from build123d import *

# Parameters (mm, degrees)
SKETCH_2_W                       = 64.02174429
SKETCH_2_H                       = 9.248919907
CUT_EXTRUDE_1_DEPTH              = 49
HOLE_WIZARD_M4_2_D               = 3.3
HOLE_WIZARD_M4_2_DEPTH           = 5.5
HOLE_WIZARD_M4_2_TIP             = 0.991420021
HOLE_WIZARD_M6_2_D               = 5
HOLE_WIZARD_M6_2_DEPTH           = 5.5
HOLE_WIZARD_M6_2_TIP             = 1.502151548
HOLE_WIZARD_M4_3_D               = 3.3
HOLE_WIZARD_M4_3_DEPTH           = 13.4
HOLE_WIZARD_M4_3_TIP             = 0.991420021
HOLE_WIZARD_M4_3_ON_FACE_2_D     = 3.3
HOLE_WIZARD_M4_3_ON_FACE_2_DEPTH = 13.4
HOLE_WIZARD_M4_3_ON_FACE_2_TIP   = 0.991420021


with BuildPart() as part:
    # 草图1 → 旋转1 (revolve)
    with BuildSketch(Plane(origin=(0, 0, 0), x_dir=(1, 0, 0), z_dir=(0, 1, 0)), mode=Mode.PRIVATE) as revolve_1_sk:
        Polygon((34.5, 7.5), (34.5, -7.5), (25.4, -7.5), (25.4, -4), (26.5, -4), (26.5, 4), (25.4, 4), (25.4, 7.5), align=None)
    revolve(revolve_1_sk.sketch.rotate(Axis((0, 0, -31.9390681), (0, 0, 1)), 180), axis=Axis((0, 0, -31.9390681), (0, 0, 1)))  # turned: the seam where the file's is

    # 草图2 → 切除-拉伸1 (cut)
    with BuildSketch(Plane.XY.offset(7.5)):
        with Locations((-1.141100508, 38.424459954)):
            Rectangle(SKETCH_2_W, SKETCH_2_H)
        with Locations((-1.141100508, -38.424459954)):
            Rectangle(SKETCH_2_W, SKETCH_2_H)
    extrude(amount=-CUT_EXTRUDE_1_DEPTH, mode=Mode.SUBTRACT)

    # M4 螺纹孔2
    with Locations(Plane(origin=(0, 33.8, 0), x_dir=(1, 0, 0), z_dir=(0, 1, 0))):
        with Locations((0, 0)):
            Hole(HOLE_WIZARD_M4_2_D / 2, depth=HOLE_WIZARD_M4_2_DEPTH)
            with Locations((0, 0, -(HOLE_WIZARD_M4_2_DEPTH + HOLE_WIZARD_M4_2_TIP / 2))):  # 118° drill point
                Cone(0, HOLE_WIZARD_M4_2_D / 2, HOLE_WIZARD_M4_2_TIP, mode=Mode.SUBTRACT)

    # M6 螺纹孔2
    with Locations(Plane(origin=(0, -33.8, 0), x_dir=(-1, 0, 0), z_dir=(0, -1, 0))):
        with Locations((0, 0)):
            Hole(HOLE_WIZARD_M6_2_D / 2, depth=HOLE_WIZARD_M6_2_DEPTH)
            with Locations((0, 0, -(HOLE_WIZARD_M6_2_DEPTH + HOLE_WIZARD_M6_2_TIP / 2))):  # 118° drill point
                Cone(0, HOLE_WIZARD_M6_2_D / 2, HOLE_WIZARD_M6_2_TIP, mode=Mode.SUBTRACT)

    # M4 螺纹孔3
    with Locations(Plane(origin=(29.877876431, 17.25, 0), x_dir=(-0.5, 0.866025404, 0), z_dir=(0.866025404, 0.5, 0))):
        with Locations((0, 0)):
            Hole(HOLE_WIZARD_M4_3_D / 2, depth=HOLE_WIZARD_M4_3_DEPTH)
            with Locations((0, 0, -(HOLE_WIZARD_M4_3_DEPTH + HOLE_WIZARD_M4_3_TIP / 2))):  # 118° drill point
                Cone(0, HOLE_WIZARD_M4_3_D / 2, HOLE_WIZARD_M4_3_TIP, mode=Mode.SUBTRACT)

    # M4 螺纹孔3 on face 2
    with Locations(Plane(origin=(-29.877876431, 17.25, 0), x_dir=(-0.500000175, -0.866025303, 0), z_dir=(-0.866025303, 0.500000175, 0))):
        with Locations((0, 0)):
            Hole(HOLE_WIZARD_M4_3_ON_FACE_2_D / 2, depth=HOLE_WIZARD_M4_3_ON_FACE_2_DEPTH)
            with Locations((0, 0, -(HOLE_WIZARD_M4_3_ON_FACE_2_DEPTH + HOLE_WIZARD_M4_3_ON_FACE_2_TIP / 2))):  # 118° drill point
                Cone(0, HOLE_WIZARD_M4_3_ON_FACE_2_D / 2, HOLE_WIZARD_M4_3_ON_FACE_2_TIP, mode=Mode.SUBTRACT)


solid = part.part
For this review, take the finished solid that the model builds, in its own axes (mm). A direction names the side the tool comes from. Coordinates: 2 decimals unless noted, no trailing zeros. Order: outer loops, then holes, each group sorted by start corner. A loop starts at its lowest first (then second) coordinate and runs counter-clockwise, first axis right, second up. Notation, with made-up numbers: (-23.75, -4.5) - (-12.75, -4.5) arc R14 cw to (-12.75, 17.5) - close; hole circle Ø8 at (-3.75, 45.25). An arc over 180 degrees is marked (long way). Answer as CSV lines item,"result". Start each with the question number.
1) To check wall thickness, follow line 1 along Y through (x, z) = (0, 6.7); line 2 along Y through (x, z) = (15.5, 5.5). State the ranges of each line that lie inside material, in increasing order. Write a range as [from, to].
2) Draft analysis for pull direction Y (two halves, no side actions). For faces 1 (the flat face through (0, 33.8, 2)), 2 (the cylindrical face through (1.216, 31.012, -1.115)), 3 (the cylindrical face through (-11.721, 22.534, 5.726)), state which applies: +Y half, -Y half, draft (parallel to the pull), parting line (faces both ways), or undercut.
3) Machinability: for faces 4 (the cylindrical face through (3.45, -26.274, -0.056)), 5 (the cylindrical face through (-0.54, -31.01, 2.44)), 6 (the cylindrical face through (34.494, -0.661, 0.105)), which of the approach directions +Z, -Z, +X, -X, +Y, -Y give a long, thin tool a straight path to every point of the face, cutting with its end or side? Answer none if there is none.
4) Insertion check: P1, Ø1.5, axis at y = 9.5, z = -2, coming from the +X side; P2, Ø4, axis at y = 21.5, z = 5.5, coming from the +X side; P3, Ø3, axis at x = 0, z = 0, coming from the -Y side. Each pin has a flat end and moves straight along its axis. Give the tip position at first contact, or say it passes through.
5) Add section B-B (x = -13.5). State the section outline as (y, z) points, then the cut area to 3 significant figures.
6) Add section A-A (y = 0). State the section outline as (x, z) points, then the cut area to 3 significant figures.
Result:
1,line 1,"[-33.8, -25.4], [25.4, 33.8]"
1,line 2,"[-30.82, -20.12], [20.12, 30.82]"
2,face 1,"+Y half"
2,face 2,"draft"
2,face 3,"undercut"
3,face 4,"none"
3,face 5,"-Y"
3,face 6,"+Z, -Z, +X"
4,P1,"x = 33.37"
4,P2,"x = 28.46"
4,P3,"y = -27.7"
5,outline,"(-31.75, -7.5) - (-21.52, -7.5) - (-21.52, -4) - (-22.8, -4) - (-22.8, 4) - (-21.52, 4) - (-21.52, 7.5) - (-31.75, 7.5) - close; (21.52, -7.5) - (31.75, -7.5) - (31.75, 7.5) - (21.52, 7.5) - (21.52, 4) - (22.8, 4) - (22.8, -4) - (21.52, -4) - close"
5,area,"286 mm^2"
6,outline,"(-34.5, -7.5) - (-25.4, -7.5) - (-25.4, -4) - (-26.5, -4) - (-26.5, 4) - (-25.4, 4) - (-25.4, 7.5) - (-34.5, 7.5) - close; (25.4, -7.5) - (34.5, -7.5) - (34.5, 7.5) - (25.4, 7.5) - (25.4, 4) - (26.5, 4) - (26.5, -4) - (25.4, -4) - close"
6,area,"255 mm^2"
